For this review, take the finished solid that the model builds, in its own axes (mm). A direction names the side the tool comes from. Round coordinates to 2 decimals unless told otherwise and drop trailing zeros. Order: outer loops, then holes, each group sorted by start corner. A loop starts at its lowest first (then second) coordinate and runs counter-clockwise, first axis right, second up. Notation, with made-up numbers: M 25,71 L 62,71 A13 cw 62,91 Z; hole C 23.5,20 d3. An arc over 180 degrees is marked long. Answer in a Markdown table with one row per item. Add a question column.
Autodesk Inventor part; units mm, degrees
ref_plane "YZ Plane" through (0, 0, 0) normal (1, 0, 0) x (0, 1, 0)
ref_plane "XZ Plane" through (0, 0, 0) normal (0, 1, 0) x (-1, 0, 0)
ref_plane "XY Plane" through (0, 0, 0) normal (0, 0, 1) x (1, 0, 0)
sketch "Sketch1" plane through (0, 0, 0) normal (0, 0, 1) x (1, 0, 0)
  line L0 (0, 0) -> (22, 0)
  line L1 (22, 0) -> (22, -20)
  line L2 (22, -20) -> (0, -20)
  line L3 (0, -20) -> (0, 0)
  line L4 (3, 0) -> (19, 0)
  line L5 (19, 0) -> (19, -17)
  line L6 (19, -17) -> (3, -17)
  line L7 (3, -17) -> (3, 0)
  dimension "d0" = 22
  dimension "d1" = 20
  dimension "d2" = 3
  dimension "d3" = 3
  dimension "d4" = 3
extrude "Extrusion1" add sketch "Sketch1" along normal blind 20 contours L0 L7 L6 L5 L1 L2 L3
sketch "Sketch4" plane through (3, -17, 0) normal (1, 0, 0) x (0, 0, -1)
  line L0 (-20, 0) -> (-20, 17)
  line L1 (0, 0) -> (-20, 0)
  line L2 (-20, 0) -> (-20, 17)
  line L3 (-20, 17) -> (0, 17)
  line L4 (0, 17) -> (0, 0)
  point P0 (0, 17)
extrude "Extrusion4" cut sketch "Sketch4" against normal through all
sketch "Sketch5" plane through (0, 0, 0) normal (0, 0, -1) x (-1, 0, 0)
  line L0 (0, -20) -> (-22, -20)
  line L1 (0, -20) -> (-4, -20)
  line L2 (-4, -20) -> (-4, -30)
  line L3 (-4, -30) -> (0, -30)
  line L4 (0, -30) -> (0, -20)
  point P0 (0, 0)
  dimension "d17" = 4
  dimension "d18" = 10
extrude "Extrusion5" add sketch "Sketch5" against normal blind 20
sketch "Sketch6" plane through (4, -30, 0) normal (1, 0, 0) x (0, 0, -1)
  line L0 (0, 10) -> (-20, 10)
  line L1 (0, 10) -> (0, 0)
  circle A0 centre (-10, 5) radius 2.5
  point P0 (0, 30)
  dimension "d21" = 5
  dimension "d22" = 10
  dimension "d23" = 5
extrude "Extrusion6" cut sketch "Sketch6" against normal through all
sketch "Sketch7" plane through (0, 0, 0) normal (0, 0, -1) x (-1, 0, 0)
  line L0 (-4, -20) -> (-22, -20)
  line L1 (-4, -30) -> (-4, -20)
  line L2 (-9, -20) -> (-4, -25)
  point P0 (0, 0)
  dimension "d26" = 5
  dimension "d27" = 5
extrude "Extrusion7" add sketch "Sketch7" against normal blind 4
sketch "Sketch8" plane through (0, 0, 20) normal (0, 0, 1) x (1, 0, 0)
  line L0 (4, -20) -> (22, -20)
  line L1 (4, -30) -> (4, -20)
  line L2 (9, -20) -> (4, -25)
  point P0 (0, 0)
  dimension "d30" = 5
  dimension "d31" = 5
extrude "Extrusion8" add sketch "Sketch8" against normal blind 4
sketch "Sketch9" plane through (19, -17, 0) normal (-1, 0, 0) x (0, 0, 1)
  line L0 (0, 17) -> (0, 0)
  line L1 (0, 0) -> (20, 0)
  circle A0 centre (10, 6) radius 1.5
  dimension "d34" = 10
  dimension "d35" = 6
  dimension "d36" = 3
extrude "Extrusion9" cut sketch "Sketch9" against normal through all
equation "\"d3\" = d2"
equation "\"d4\" = d2"
equation "\"d27\" = d26"
equation "\"d30\" = d26"
equation "\"d31\" = d30"
properties part number "LED strip mount v04"
1. For faces 1 (the flat face through (5, -21, 4)), 2 (the flat face through (10, -17, 10)), 3 (the flat face through (7, -22, 2)), list the 3-axis set-ups (+Z, -Z, +X, -X, +Y, -Y) from which the entire face can be reached by the end or side of a thin tool; tool diameter is ignored.
2. Clearance check with flat-ended pins moving along their axes: pin 1 Ø10 at (x, z) = (10, 9) entering from +Y; pin 2 Ø5.5 at (x, z) = (13, 7) entering from -Y; pin 3 Ø8 at (x, y) = (18, -13.5) entering from +Z; pin 4 Ø8 at (y, z) = (-25, 9) entering from +X. State where each tip first meets the part, or that it passes through.
3. Consider section D-D on z = 3. Write out the cut boundary in (x, y).
4. To check wall thickness, follow probe 1 along Y at (x, z) = (20.35, 10); probe 2 along X at (y, z) = (-8.25, 1.5); probe 3 along Y at (x, z) = (12.25, 1). State the ranges of each line that lie inside material, in increasing order. Write a range as [from, to].
5. The part is to be moulded in two halves that separate along Y. For faces 4 (the flat face through (19, -8, 10)), 5 (the cylindrical face through (20.5, -11.9, 8.8)), 6 (the flat face through (2, -30, 10)), say which applies: pulls with the +Y half, pulls with the -Y half, needs draft (parallel to the pull), parting line crosses it, or undercut.
6. Consider section C-C on x = 5.25. Write out the cut boundary in (y, z), plus the area to 3 significant figures.
7. Consider section A-A on y = -11. Write out the cut boundary in (x, z).
8. Consider section B-B on z = 10. Write out the cut boundary in (x, y), plus the area to 3 significant figures.
Solved:
| question | item | result |
|---|---|---|
| 1 | face 1 | +X, -Y |
| 1 | face 2 | +Z, -Z, -X, +Y |
| 1 | face 3 | +Z, -Z, +X, -Y |
| 2 | pin 1 | stops at y = -17 |
| 2 | pin 2 | stops at y = -20 |
| 2 | pin 3 | stops at z = 20 |
| 2 | pin 4 | stops at x = 4 |
| 3 | outline | M 0,-30 L 4,-30 L 4,-25 L 9,-20 L 22,-20 L 22,0 L 19,0 L 19,-17 L 0,-17 Z |
| 4 | probe 1 | y = [-20, -12.5], [-9.5, 0] |
| 4 | probe 2 | x = [19, 22] |
| 4 | probe 3 | y = [-20, -17] |
| 5 | face 4 | needs draft |
| 5 | face 5 | undercut |
| 5 | face 6 | pulls with the -Y half |
| 6 | outline | M -23.75,0 L -17,0 L -17,20 L -23.75,20 L -23.75,16 L -20,16 L -20,4 L -23.75,4 Z |
| 6 | area | 90.0 mm^2 |
| 7 | outline | M 19,0 L 22,0 L 22,8.5 L 19,8.5 Z; M 19,11.5 L 22,11.5 L 22,20 L 19,20 Z |
| 8 | outline | M 0,-30 L 4,-30 L 4,-27.5 L 0,-27.5 Z; M 0,-22.5 L 4,-22.5 L 4,-20 L 22,-20 L 22,-12.5 L 19,-12.5 L 19,-17 L 0,-17 Z; M 19,-9.5 L 22,-9.5 L 22,0 L 19,0 Z |
| 8 | area | 128 mm^2 |
